from build123d import *

# Parameters (mm, degrees)
PAD_DEPTH       = 20
SKETCH004_R     = 2
POCKET002_DEPTH = 185.001
SKETCH005_R     = 2
POCKET003_DEPTH = 85.001


with BuildPart() as part:
    # Sketch → Pad (new body)
    with BuildSketch(Plane.XY):
        Polygon((-10, -42.5), (175, -42.5), (175, -30.5), (0, -30.5), (0, 30.5), (175, 30.5), (175, 42.5), (-10, 42.5), (-10, 38.5), (-17, 38.5), (-17, 33.5), (-10, 33.5), (-10, -33.5), (-17, -33.5), (-17, -38.5), (-10, -38.5), align=None)
    extrude(amount=PAD_DEPTH)

    # Sketch004 → Pocket002 (cut, through all)
    with BuildSketch(Plane(origin=(-10, 0, 0), x_dir=(0, -1, 0), z_dir=(-1, 0, 0))):
        with Locations((0, 10)):
            Circle(SKETCH004_R)
    extrude(amount=-POCKET002_DEPTH, mode=Mode.SUBTRACT)

    # Sketch005 → Pocket003 (cut, through all)
    with BuildSketch(Plane.XZ.offset(42.5)):
        with Locations((-5, 10)):
            Circle(SKETCH005_R)
        with Locations((165, 10)):
            Circle(SKETCH005_R)
    extrude(amount=-POCKET003_DEPTH, mode=Mode.SUBTRACT)


solid = part.part
CAD build for the part. Positions are in the model's coordinates, mm. A direction names the side the tool comes from. Round coordinates to 2 decimals unless told otherwise and drop trailing zeros. Order: outer loops, then holes, each group sorted by start corner. A loop starts at its lowest first (then second) coordinate and runs counter-clockwise, first axis right, second up. Notation, with made-up numbers: M -30.75,73 L 22.25,73 A21 ccw 22.25,84 Z; hole C -8.75,48.25 d1. An arc over 180 degrees is marked long. Use one line per item in the form item = value.
Q1. Saw through at A-A on x = 96.5. Give the cut face in (y, z).
Recorded:
outline = M -42.5,0 L -30.5,0 L -30.5,20 L -42.5,20 Z; M 30.5,0 L 42.5,0 L 42.5,20 L 30.5,20 Z
Q2. Flat gauge pins, fed straight in: P1, Ø10, axis at y = 12.5, z = 7, coming from the +X side; P2, Ø5.5, axis at x = -13, z = 12.5, coming from the -Y side; P3, Ø7.5, axis at x = -15, z = 6, coming from the +Y side. Where does each tip first touch, or does it go through?
Recorded:
P1 = 0
P2 = -38.5
P3 = 38.5
Q3. Two-plate mould, pull along Y, no slides. Class faces 1 (the flat face through (0, -0.4, 7.6)), 2 (the flat face through (86, 32, 20)), 3 (the flat face through (-13, 38.5, 10)): +Y half, -Y half, draft (parallel to the pull), parting line (faces both ways), or undercut.
Recorded:
face_1 = undercut
face_2 = draft
face_3 = +Y half
Q4. Saw through at D-D on y = 20. Give the cut face in (x, z).
Recorded:
outline = M -10,0 L 0,0 L 0,20 L -10,20 Z; hole C -5,10 d4
Q5. Saw through at B-B on z = 6. Give the cut face in (x, y).
Recorded:
outline = M -17,-38.5 L -10,-38.5 L -10,-42.5 L 175,-42.5 L 175,-30.5 L 0,-30.5 L 0,30.5 L 175,30.5 L 175,42.5 L -10,42.5 L -10,38.5 L -17,38.5 L -17,33.5 L -10,33.5 L -10,-33.5 L -17,-33.5 Z
Q6. Saw through at C-C on x = 165. Give the cut face in (y, z), then the cut area to 3 significant figures.
Recorded:
outline = M -42.5,0 L -30.5,0 L -30.5,8 L -42.5,8 Z; M -42.5,12 L -30.5,12 L -30.5,20 L -42.5,20 Z; M 30.5,0 L 42.5,0 L 42.5,8 L 30.5,8 Z; M 30.5,12 L 42.5,12 L 42.5,20 L 30.5,20 Z
area = 384 mm^2
Q7. Probe L1, parallel to X at y = -38, z = 9.75; L2, parallel to Y at x = 11, z = 7.75; L3, parallel to X at y = 30, z = 10. List the from-to ranges inside material, lowest first.
Recorded:
L1 = -17 to -6.98, -3.02 to 163.02, 166.98 to 175
L2 = -42.5 to -30.5, 30.5 to 42.5
L3 = -10 to -7, -3 to 0
Q8. Which spindle directions (+Z, -Z, +X, -X, +Y, -Y) get a long thin tool onto all of the face, cutting with end or side? Do faces 4 (the flat face through (-14, -38.5, 10)), 5 (the flat face through (-13, -33.5, 10)), 6 (the flat face through (89, -30.5, 10)). Say none if no direction does.
Recorded:
face_4 = +Z, -Z, -X, -Y
face_5 = +Z, -Z, -X
face_6 = +Z, -Z, +X
